Part model, mm, in its own coordinate system. A direction names the side the tool comes from. Give positions to 0.01 mm unless a question says otherwise; leave off trailing zeros. Write each loop counter-clockwise with the first axis right and the second up, starting at its lowest first coordinate (ties: lowest second). Pieces come first, ordered by that corner, then holes.
```python
from build123d import *

# Parameters (mm, degrees)
SKETCH_W        = 49
SKETCH_H        = 18
PAD_DEPTH       = 2
PAD001_DEPTH    = 21
SKETCH002_W     = 10
SKETCH002_H     = 21
POCKET_DEPTH    = 2
SKETCH003_W     = 10
SKETCH003_H     = 21
POCKET001_DEPTH = 2
FILLET_R        = 3
FILLET001_R     = 3
FILLET002_R     = 2
FILLET003_R     = 2
FILLET004_R     = 2
FILLET005_R     = 2
SKETCH004_W     = 9
SKETCH004_H     = 9
PAD002_DEPTH    = 6
FILLET006_R     = 5


with BuildPart() as part:
    # Sketch → Pad (new body)
    with BuildSketch(Plane.XY):
        with Locations((24.5, 9)):
            Rectangle(SKETCH_W, SKETCH_H)
    extrude(amount=PAD_DEPTH)

    # Sketch001 (on Face6 of Pad) → Pad001 (join)
    with BuildSketch(Plane.XY.offset(2)):
        Polygon((2, 18), (2, 2), (47, 2), (47, 18), (49, 18), (49, 0), (0, 0), (0, 18), align=None)
    extrude(amount=PAD001_DEPTH)

    # Sketch002 (on Face5 of Pad001) → Pocket (cut)
    with BuildSketch(Plane.XZ):
        with Locations((10, 12.5)):
            Rectangle(SKETCH002_W, SKETCH002_H)
    extrude(amount=-POCKET_DEPTH, mode=Mode.SUBTRACT)

    # Sketch003 (on Face7 of Pocket) → Pocket001 (cut)
    with BuildSketch(Plane.XZ):
        with Locations((39, 12.5)):
            Rectangle(SKETCH003_W, SKETCH003_H)
    extrude(amount=-POCKET001_DEPTH, mode=Mode.SUBTRACT)

    # Fillet
    fillet_edges = [part.edges().sort_by_distance(p)[0] for p in [
        (1, 18, 23),
    ]]
    fillet(fillet_edges, radius=FILLET_R)

    # Fillet001
    fillet001_edges = [part.edges().sort_by_distance(p)[0] for p in [
        (48, 18, 23),
    ]]
    fillet(fillet001_edges, radius=FILLET001_R)

    # Fillet002
    fillet002_edges = [part.edges().sort_by_distance(p)[0] for p in [
        (5, 1, 23),
    ]]
    fillet(fillet002_edges, radius=FILLET002_R)

    # Fillet003
    fillet003_edges = [part.edges().sort_by_distance(p)[0] for p in [
        (15, 1, 23),
    ]]
    fillet(fillet003_edges, radius=FILLET003_R)

    # Fillet004
    fillet004_edges = [part.edges().sort_by_distance(p)[0] for p in [
        (34, 1, 23),
    ]]
    fillet(fillet004_edges, radius=FILLET004_R)

    # Fillet005
    fillet005_edges = [part.edges().sort_by_distance(p)[0] for p in [
        (44, 1, 23),
    ]]
    fillet(fillet005_edges, radius=FILLET005_R)

    # Sketch004 (on Face15 of Fillet005) → Pad002 (join)
    with BuildSketch(Plane(origin=(0, 2, 0), x_dir=(-1, 0, 0), z_dir=(0, 1, 0))):
        with Locations((-24.5, 6.5)):
            Rectangle(SKETCH004_W, SKETCH004_H)
    extrude(amount=PAD002_DEPTH)

    # Fillet006
    fillet006_edges = [part.edges().sort_by_distance(p)[0] for p in [
        (24.5, 8, 11),
    ]]
    fillet(fillet006_edges, radius=FILLET006_R)


solid = part.part
```
1) Saw through at B-B, the plane y = 6. Write the cut outline in (x, z).
Answers follow:
outline: (0, 0) - (49, 0) - (49, 23) - (47, 23) - (47, 2) - (29, 2) - (29, 10) - (20, 10) - (20, 2) - (2, 2) - (2, 23) - (0, 23) - close
2) Pin check, flat tips, straight feed: pin 1 Ø12 at (x, z) = (14.5, 4.5) entering from +Y; pin 2 Ø0.9 at (x, z) = (3.5, 13) entering from +Y; pin 3 Ø1.2 at (x, z) = (23, 3.5) entering from +Y; pin 4 Ø1.5 at (x, y) = (41, 12) entering from +Z. Stop position of each tip, or through.
Answers follow:
pin 1: stops at y = 18
pin 2: stops at y = 2
pin 3: stops at y = 8
pin 4: stops at z = 2
3) Two-plate mould, pull along X, no slides. Class faces 4 (the face through (49, 9, 11)), 5 (the face through (0, 9, 11)), 6 (the face through (1, 8, 23)), 7 (the face through (15.57, 1.01, 22.4)): +X half, -X half, draft (parallel to the pull), parting line (faces both ways), or undercut.
Answers follow:
face 4: +X half
face 5: -X half
face 6: draft
face 7: undercut
4) Wall check: L1, parallel to X at y = 17.25, z = 5; L2, parallel to X at y = 7.5, z = 6; L3, parallel to Z at x = 19.5, y = 14.25. Give the ranges that are in metal, low to high.
Answers follow:
L1: x = 0 to 2, 47 to 49
L2: x = 0 to 2, 20 to 29, 47 to 49
L3: z = 0 to 2
5) 3-axis set-ups, long thin cutter, end or side, ignore diameter. For faces 1 (the face through (29, 5, 6)), 2 (the face through (44.57, 1.01, 22.4)), 3 (the face through (1.01, 17.14, 22.1)): which of +Z, -Z, +X, -X, +Y, -Y reach the whole face in a straight line?
Answers follow:
face 1: +Z, +Y
face 2: +Z, +Y, -Y
face 3: +Z, +X, -X, +Y
6) Saw through at A-A, the plane z = 3. Write the cut outline in (x, y), then the cut area to 3 significant figures.
Answers follow:
outline: (0, 0) - (5, 0) - (5, 2) - (2, 2) - (2, 18) - (0, 18) - close; (15, 0) - (34, 0) - (34, 2) - (29, 2) - (29, 8) - (20, 8) - (20, 2) - (15, 2) - close; (44, 0) - (49, 0) - (49, 18) - (47, 18) - (47, 2) - (44, 2) - close
area: 176 mm2
7) Saw through at D-D, the plane z = 14.25. Write the cut outline in (x, y), then the cut area to 3 significant figures.
Answers follow:
outline: (0, 0) - (5, 0) - (5, 2) - (2, 2) - (2, 18) - (0, 18) - close; (15, 0) - (34, 0) - (34, 2) - (15, 2) - close; (44, 0) - (49, 0) - (49, 18) - (47, 18) - (47, 2) - (44, 2) - close
area: 122 mm2
8) Saw through at C-C, the plane x = 17.5. Write the cut outline in (y, z), then the cut area to 3 significant figures.
Answers follow:
outline: (0, 0) - (18, 0) - (18, 2) - (2, 2) - (2, 23) - (0, 23) - close
area: 78.0 mm2
